Could you check a few things on this model? Use its own coordinates, in mm. Give positions to 0.01 mm unless a question says otherwise; leave off trailing zeros. Loops run counter-clockwise (first coordinate to the right, second up) from the corner with the lowest first, then second, coordinate; pieces in that order, holes last. Notation, with made-up numbers: M -4,-10.5 L 16,-10.5 A14 cw 16,-3.5 Z; hole C 55,-2 d10. An arc over 180 degrees is marked long. Answer in a Markdown table with one row per item. Add a question column.
1. If we section it at C-C on z = 2: Count the separate pieces of the cut face and the enclosed holes in it, then the cut area to 3 significant figures.
2. If we section it at B-B on x = 0: List the corners of the cut face in (y, z) for me, then the cut area to 3 significant figures.
3. I need wall thicknesses on line 1 along X through (y, z) = (-8.5, 2.75); line 2 along X through (y, z) = (-7.5, 3.35); line 3 along Y through (x, z) = (-5, 1.6). Which ranges of each line are inside material? Lowest first, please. Write a range as from..to.
4. If we section it at A-A on y = 0: List the corners of the cut face in (x, z) for me, then the cut area to 3 significant figures.
5. If we section it at D-D on x = -10: List the corners of the cut face in (y, z) for me.
6. I'm going to push flat-ended pins straight in: pin 1 Ø2.5 at (x, y) = (5, 8.66) entering from +Z; pin 2 Ø4.5 at (x, y) = (21, 0) entering from -Z; pin 3 Ø1.5 at (y, z) = (18.5, 1.5) entering from -X; pin 4 Ø5 at (x, y) = (0, -21) entering from -Z. Where does each tip first touch, or does it pass through?
```python
from build123d import *

# Parameters (mm, degrees)
SKETCH_1_R          = 27
EXTRUDE_1_DEPTH     = 4
SKETCH_2_R          = 1.5
SKETCH_2_R_2        = 2
CUT_EXTRUDE_1_DEPTH = 10
CHAMFER_1_SIZE      = 1


with BuildPart() as part:
    # 草图1 → 凸台-拉伸1 (new body)
    with BuildSketch(Plane.XY):
        Circle(SKETCH_1_R)
    extrude(amount=EXTRUDE_1_DEPTH)

    # 草图2 → 切除-拉伸1 (cut)
    with BuildSketch(Plane.XY.offset(4)):
        with Locations((5, 8.660254038)):
            Circle(SKETCH_2_R)
        with Locations((10, 0)):
            Circle(SKETCH_2_R)
        with Locations((5, -8.660254038)):
            Circle(SKETCH_2_R)
        with Locations((-5, -8.660254038)):
            Circle(SKETCH_2_R)
        with Locations((-10, 0)):
            Circle(SKETCH_2_R)
        with Locations((-5, 8.660254038)):
            Circle(SKETCH_2_R)
        with Locations((0, 21)):
            Circle(SKETCH_2_R_2)
        with Locations((21, 0)):
            Circle(SKETCH_2_R_2)
        with Locations((0, -21)):
            Circle(SKETCH_2_R_2)
        with Locations((-21, 0)):
            Circle(SKETCH_2_R_2)
    extrude(amount=-CUT_EXTRUDE_1_DEPTH, mode=Mode.SUBTRACT)

    # 倒角1
    chamfer_1_edges = [part.edges().sort_by_distance(p)[0] for p in [
        (-23, 0, 0),
        (-2, 21, 0),
        (19, 0, 0),
        (-2, -21, 0),
    ]]
    chamfer(chamfer_1_edges, length=CHAMFER_1_SIZE)


solid = part.part
```
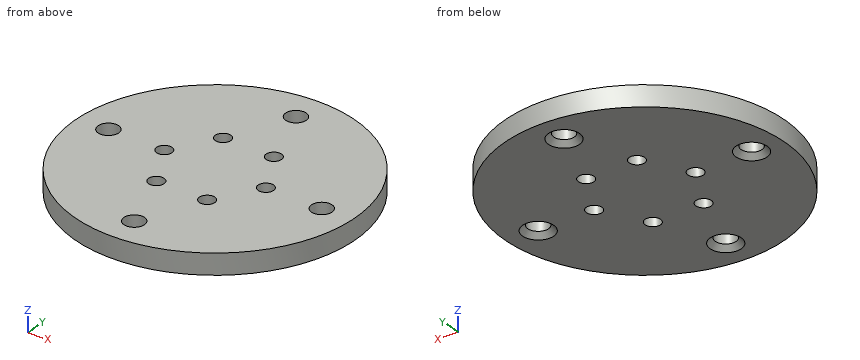
Results:
| question | item | result |
|---|---|---|
| 1 | separate pieces | 1 |
| 1 | enclosed holes | 10 |
| 1 | area | 2,200 mm2 |
| 2 | outline | M -27,0 L -24,0 L -23,1 L -23,4 L -27,4 Z; M -19,1 L -18,0 L 18,0 L 19,1 L 19,4 L -19,4 Z; M 23,1 L 24,0 L 27,0 L 27,4 L 23,4 Z |
| 2 | area | 182 mm2 |
| 3 | line 1 | -25.63..-6.49, -3.51..3.51, 6.49..25.63 |
| 3 | line 2 | -25.94..-5.95, -4.05..4.05, 5.95..25.94 |
| 3 | line 3 | -26.53..-10.16, -7.16..7.16, 10.16..26.53 |
| 4 | outline | M -27,0 L -24,0 L -23,1 L -23,4 L -27,4 Z; M -19,1 L -18,0 L -11.5,0 L -11.5,4 L -19,4 Z; M -8.5,0 L 8.5,0 L 8.5,4 L -8.5,4 Z; M 11.5,0 L 18,0 L 19,1 L 19,4 L 11.5,4 Z; M 23,1 L 24,0 L 27,0 L 27,4 L 23,4 Z |
| 4 | area | 158 mm2 |
| 5 | outline | M -25.08,0 L -1.5,0 L -1.5,4 L -25.08,4 Z; M 1.5,0 L 25.08,0 L 25.08,4 L 1.5,4 Z |
| 6 | pin 1 | through |
| 6 | pin 2 | z = 0.75 |
| 6 | pin 3 | x = -20.35 |
| 6 | pin 4 | z = 0.5 |
